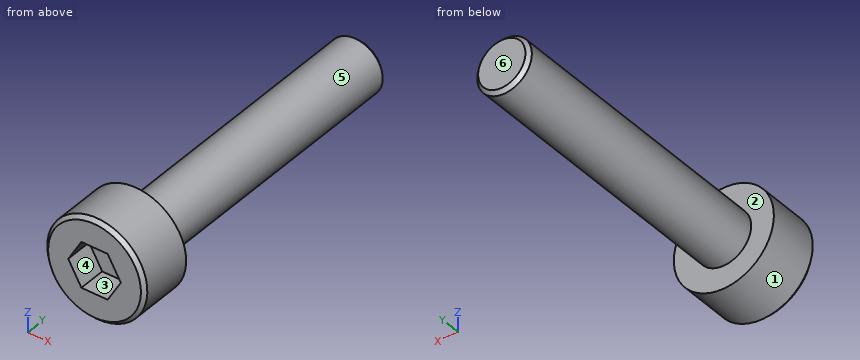
from build123d import *

# Parameters (mm, degrees)
SIMPLIFIED_START                    = -3
SIMPLIFIED_NOMINAL_HEX_SOCKET_DEPTH = 1.5


with BuildPart() as part:
    # Reconstructed nominal axial profile → Native revolved geometry (revolve)
    with BuildSketch(Plane.XY, mode=Mode.PRIVATE) as native_revolved_geometry_sk:
        Polygon((0, -3), (2.55, -3), (2.75, -2.8), (2.75, 0), (1.5, 0), (1.5, 15.8), (1.3, 16), (0, 16), align=None)
    revolve(native_revolved_geometry_sk.sketch.rotate(Axis((0, -500, 0), (0, 1, 0)), 90), axis=Axis((0, -500, 0), (0, 1, 0)))

    # Sketch2 → Simplified nominal hex socket (cut)
    with BuildSketch(Plane(origin=(0, 0, 0), x_dir=(1, 0, 0), z_dir=(0, 1, 0)).offset(SIMPLIFIED_START)):
        Polygon((1.443375673, 0), (0.721687836, -1.25), (-0.721687836, -1.25), (-1.443375673, 0), (-0.721687836, 1.25), (0.721687836, 1.25), align=None)
    extrude(amount=SIMPLIFIED_NOMINAL_HEX_SOCKET_DEPTH, mode=Mode.SUBTRACT)


solid = part.part
Can you work these out from the model? Positions are in its coordinate system, mm. Face numbers are marked on the shaded views. A direction names the side the tool comes from. Coordinates: 2 decimals unless noted, no trailing zeros. Loops run counter-clockwise (first coordinate to the right, second up) from the corner with the lowest first, then second, coordinate; pieces in that order, holes last. Notation, with made-up numbers: (14.25, 29.5) - (63.25, 29.5) arc R20 ccw to (63.25, 65.5) - close; hole circle Ø1 at (-9, 29). An arc over 180 degrees is marked (long way). Put each result on its own line as item: value. Start each with the question number.
Item 1: Suppose I cut it at A-A (x = 0). Please give me the cut outline in (y, z), and give its area (3 significant figures).
Item 2: For pin 1 (2 mm diameter, centred on x = 0, y = 13.5, fed in from -Z); pin 2 (2 mm diameter, centred on x = 0, y = 13, fed in from +Z), each with a flat end and sliding along its axis, tell me the tip position at first contact or that it passes through.
Item 3: If I drill on line 1 along Y through (x, z) = (-1.15, -1.9); line 2 along Y through (x, z) = (-0.1, 0.1); line 3 along Z through (x, y) = (0.05, 10.5), over which ranges is the centre line in solid material (lowest first)?
Item 4: Suppose I cut it at B-B (y = -1). Please give me the cut outline in (x, z).
Item 5: Which directions (+Z, -Z, +X, -X, +Y, -Y) give clear straight access to the entire face, cutting with the end or side of a thin tool? Please do the marked faces 4, 5 and 6.
Item 6: If we mould it in two halves opening along X, with no side actions, what happens to the marked faces 1, 2 and 3? For each: +X half, -X half, draft (parallel to the pull), parting line (faces both ways), or undercut.
Item 7: Suppose I cut it at C-C (y = 10). Please give me the cut outline in (x, z), and give its area (3 significant figures).
Here are the results:
1. outline: (-3, -2.55) - (-2.8, -2.75) - (0, -2.75) - (0, -1.5) - (15.8, -1.5) - (16, -1.3) - (16, 1.3) - (15.8, 1.5) - (0, 1.5) - (0, 2.75) - (-2.8, 2.75) - (-3, 2.55) - (-3, 1.25) - (-1.5, 1.25) - (-1.5, -1.25) - (-3, -1.25) - close
1. area: 60.7 mm²
2. pin 1: z = -1.5
2. pin 2: z = 1.5
3. line 1: -3 to 0
3. line 2: -1.5 to 16
3. line 3: -1.5 to 1.5
4. outline: circle Ø5.5 at (0, 0)
5. face 4: -Y
5. face 5: +Y
5. face 6: +Z, -Z, +X, -X, +Y
6. face 1: parting line
6. face 2: draft
6. face 3: undercut
7. outline: circle Ø3 at (0, 0)
7. area: 7.07 mm²
